CAD build for the part. Positions are in the model's coordinates, mm. A direction names the side the tool comes from. Round coordinates to 2 decimals unless told otherwise and drop trailing zeros. Order: outer loops, then holes, each group sorted by start corner. A loop starts at its lowest first (then second) coordinate and runs counter-clockwise, first axis right, second up. Notation, with made-up numbers: (-32, 73.25) -> (0, 73.25) arc R20 cw to (0, 88.25) -> close; hole circle Ø7 at (12.5, -24.5). An arc over 180 degrees is marked (long way). Answer as CSV lines item,"result". Start each with the question number.
from build123d import *

# Parameters (mm, degrees)
BOSS_EXTRUDE1_DEPTH     = 20
BOSS_EXTRUDE2_DEPTH     = 20
FILLET1_R               = 3
CHAMFER1_SIZE           = 3
FILLET2_R               = 1
CUT_EXTRUDE1_DEPTH      = 71.578127074
CUT_EXTRUDE2_DEPTH      = 2
CUT_EXTRUDE2_DEPTH_BACK = 2
CUT_EXTRUDE2_START      = -10
CHAMFER2_START          = 44.201779004
CHAMFER2_OUTLINE_W      = 6
CHAMFER2_OUTLINE_H      = 20
CHAMFER2_DEPTH          = 1.294789205


with BuildPart() as part:
    # Sketch1 → Boss-Extrude1 (new body)
    with BuildSketch(Plane.XY):
        with BuildLine():
            Line((18, 45.5), (18, 41.407980081))
            Line((18, 41.407980081), (22, 41.407980081))
            Line((22, 41.407980081), (22, 50.5))
            Line((22, 50.5), (-5.5, 50.5))
            Line((-5.5, 50.5), (-5.5, 28.873187411))
            Line((-5.5, 28.873187411), (-5.5, 16.423287813))
            Line((-5.5, 16.423287813), (-0.5, 16.423287813))
            Line((-0.5, 16.423287813), (-0.5, 19))
            Line((-0.5, 19), (5, 19))
            Line((5, 19), (5, 27))
            Line((5, 27), (-0.5, 27))
            Line((-0.5, 27), (-0.5, 44))
            ThreePointArc((-0.5, 44), (-1.560660172, 46.560660172), (1, 45.5))
            Line((1, 45.5), (18, 45.5))
        make_face()
        with BuildLine():
            Line((-5.5, 16.423287813), (-5.5, 28.873187411))
            ThreePointArc((-5.5, 28.873187411), (-9.307611845, 19.680799255), (-18.5, 15.873187411))
            Line((-18.5, 15.873187411), (-21.5, 15.873187411))
            ThreePointArc((-21.5, 15.873187411), (-29.723519433, 18.660367749), (-34.557759664, 25.873187411))
            Line((-34.557759664, 25.873187411), (-39.557759664, 25.873187411))
            ThreePointArc((-39.557759664, 25.873187411), (-33.539294452, 14.749097831), (-21.5, 10.873187411))
            Line((-21.5, 10.873187411), (-18.5, 10.873187411))
            ThreePointArc((-18.5, 10.873187411), (-11.432404679, 12.31875911), (-5.5, 16.423287813))
        make_face()
    extrude(amount=-BOSS_EXTRUDE1_DEPTH)

    # Sketch4 → Boss-Extrude2 (add)
    with BuildSketch(Plane.XY):
        with BuildLine():
            Line((-5.5, 49.330303976), (-5.5, 36.880404378))
            ThreePointArc((-5.5, 36.880404378), (-9.307611845, 46.072792533), (-18.5, 49.880404378))
            Line((-18.5, 49.880404378), (-21.5, 49.880404378))
            ThreePointArc((-21.5, 49.880404378), (-29.723519433, 47.09322404), (-34.557759664, 39.880404378))
            Line((-34.557759664, 39.880404378), (-39.557759664, 39.880404378))
            ThreePointArc((-39.557759664, 39.880404378), (-33.539294452, 51.004493958), (-21.5, 54.880404378))
            Line((-21.5, 54.880404378), (-18.5, 54.880404378))
            ThreePointArc((-18.5, 54.880404378), (-11.432404679, 53.434832679), (-5.5, 49.330303976))
        make_face()
    extrude(amount=-BOSS_EXTRUDE2_DEPTH)

    # Fillet1
    # the kernel refuses this fillet: 3 mm, written as the material it takes off along each edge
    with BuildSketch(Plane(origin=(22, 41.407980081, 7.5), x_dir=(-1, 0, 0), z_dir=(0, 0, -1)), Plane(origin=(22, 50.5, 7.5), x_dir=(0, -1, 0), z_dir=(0, 0, -1))) as fillet1_piece_1:
        with BuildLine():
            CenterArc((FILLET1_R, FILLET1_R), FILLET1_R, 180, 90)
            Line((0, FILLET1_R), (-FILLET1_R * 0.02, FILLET1_R))
            Line((-FILLET1_R * 0.02, FILLET1_R), (-FILLET1_R * 0.02, -FILLET1_R * 0.02))
            Line((-FILLET1_R * 0.02, -FILLET1_R * 0.02), (FILLET1_R, -FILLET1_R * 0.02))
            Line((FILLET1_R, -FILLET1_R * 0.02), (FILLET1_R, 0))
        make_face()
    extrude(amount=35, mode=Mode.SUBTRACT)
    with BuildSketch(Plane(origin=(-5.5, 50.5, 5.942425513), x_dir=(1, 0, 0), z_dir=(0, 0, -1))) as fillet1_piece_2_section:
        with BuildLine():
            CenterArc((2.376970205, 3), FILLET1_R, 217.596829801, 52.403170199)
            Line((0, 1.169696024), (-0.047539404, 1.133089945))
            ThreePointArc((-0.047539404, 1.133089945), (-0.06, 0.584848012), (-0.06, 0))
            Line((-0.06, 0), (0, -0.06))
            Line((0, -0.06), (2.376970205, -0.06))
            Line((2.376970205, -0.06), (2.376970205, 0))
        make_face()
    fillet1_piece_2 = extrude(amount=31.884851026, mode=Mode.PRIVATE)
    fillet1_piece_2 = fillet1_piece_2 - Plane(origin=(-18.5, 36.880404378, 5.942425513), x_dir=(0, 1, 0), z_dir=(0, 0, 1)) * Cylinder(18, 74, mode=Mode.PRIVATE)
    add(fillet1_piece_2, mode=Mode.SUBTRACT)

    # Chamfer1
    chamfer1_edges = [part.edges().sort_by_distance(p)[0] for p in [
        (5, 19, -10),
    ]]
    chamfer(chamfer1_edges, length=CHAMFER1_SIZE)

    # Fillet2
    fillet2_edges = [part.edges().sort_by_distance(p)[0] for p in [
        (-0.5, 16.423287813, -10),
        (1, 45.5, -10),
        (-0.5, 44, -10),
        (-34.557759664, 39.880404378, -10),
        (-39.557759664, 39.880404378, -10),
    ]]
    fillet(fillet2_edges, radius=FILLET2_R)

    # Sketch1<3> → Cut-Extrude1 (cut, through all)
    with BuildSketch(Plane.XY):
        with BuildLine():
            Line((-34.557759664, 25.873187411), (-39.557759664, 25.873187411))
            ThreePointArc((-39.557759664, 25.873187411), (-33.539294452, 14.749097831), (-21.5, 10.873187411))
            Line((-21.5, 10.873187411), (-18.5, 10.873187411))
            ThreePointArc((-18.5, 10.873187411), (-11.432404679, 12.31875911), (-5.5, 16.423287813))
            Line((-5.5, 16.423287813), (-5.5, 28.873187411))
            ThreePointArc((-5.5, 28.873187411), (-9.307611845, 19.680799255), (-18.5, 15.873187411))
            Line((-18.5, 15.873187411), (-21.5, 15.873187411))
            ThreePointArc((-21.5, 15.873187411), (-29.723519433, 18.660367749), (-34.557759664, 25.873187411))
        make_face()
    extrude(amount=-CUT_EXTRUDE1_DEPTH, mode=Mode.SUBTRACT)

    # Sketch3 → Cut-Extrude2 (cut, two sides: drawn at the far end of the back side and taken through both)
    with BuildSketch(Plane.XY.offset(CUT_EXTRUDE2_START - CUT_EXTRUDE2_DEPTH_BACK)):
        with BuildLine():
            ThreePointArc((-10.615862632, 48.696779185), (-12.77767622, 49.881994518), (-15.111856664, 50.675578184))
            Line((-15.111856664, 50.675578184), (-14.837502866, 49.3538207))
            ThreePointArc((-14.837502866, 49.3538207), (-12.420426421, 48.371217451), (-10.248251304, 46.925733813))
            Line((-10.248251304, 46.925733813), (-10.615862632, 48.696779185))
        make_face()
        with BuildLine():
            ThreePointArc((-4.45647435, 39.017159612), (-5.14675526, 41.725731045), (-6.354052632, 44.246699113))
            Line((-6.354052632, 44.246699113), (-6.995300859, 42.933659509))
            ThreePointArc((-6.995300859, 42.933659509), (-5.87936038, 39.99800852), (-5.5, 36.880404378))
            Line((-5.5, 36.880404378), (-4.45647435, 39.017159612))
        make_face()
        with BuildLine():
            ThreePointArc((-21.5, 53.034307539), (-31.973681851, 49.335761876), (-37.80235804, 39.880404378))
            Line((-37.80235804, 39.880404378), (-35.80235804, 39.880404378))
            ThreePointArc((-35.80235804, 39.880404378), (-30.584504262, 47.950694244), (-21.5, 51.085556106))
            Line((-21.5, 51.085556106), (-18.5, 51.085556106))
            ThreePointArc((-18.5, 51.085556106), (-16.793571188, 50.982689168), (-15.111856664, 50.675578184))
            ThreePointArc((-15.111856664, 50.675578184), (-12.77767622, 49.881994518), (-10.615862632, 48.696779185))
            ThreePointArc((-10.615862632, 48.696779185), (-8.240766267, 46.705599481), (-6.354052632, 44.246699113))
            ThreePointArc((-6.354052632, 44.246699113), (-5.14675526, 41.725731045), (-4.45647435, 39.017159612))
            ThreePointArc((-4.45647435, 39.017159612), (-4.418325892, 35.011503653), (-5.5, 31.15446903))
            Line((-5.5, 31.15446903), (-5.5, 28.873187411))
            Line((-5.5, 28.873187411), (-5.5, 27.291421776))
            ThreePointArc((-5.5, 27.291421776), (-4.080428513, 44.162199863), (-18.5, 53.034307539))
            Line((-18.5, 53.034307539), (-21.5, 53.034307539))
        make_face()
    extrude(amount=CUT_EXTRUDE2_DEPTH + CUT_EXTRUDE2_DEPTH_BACK, mode=Mode.SUBTRACT)

    # Chamfer2: read off the stored shape, not the designer's step
    # Chamfer2 outline → Chamfer2 (cut)
    with BuildSketch(Plane(origin=(0, 0, 0), x_dir=(0.8164965809277286, -0.5773502691896223, 0), z_dir=(0.5773502691896223, 0.8164965809277285, 0)).offset(CHAMFER2_START)):
        with Locations((-9, 10)):
            Rectangle(CHAMFER2_OUTLINE_W, CHAMFER2_OUTLINE_H)
    extrude(amount=CHAMFER2_DEPTH, mode=Mode.SUBTRACT)


solid = part.part
Item 1: Tool access for faces 4 (the flat face through (-10.43, 47.8, -10.03)), 5 (the flat face through (-14, 50, -12)), 6 (the cylindrical face through (-9.207, 45.971, -9.86)): list every direction of +Z, -Z, +X, -X, +Y, -Y with a clear straight run to the whole face (end or side of a thin tool).
Item 2: Band-saw the part on B-B, the plane y = 34.5. Give the cut face in (x, z).
Item 3: Band-saw the part on C-C, the plane x = -29. Give the cut face in (y, z).
Item 4: Mould opens along Y. For faces 1 (the flat face through (-38, 39.88, -10)), 2 (the flat face through (5, 24, -10)), 3 (the flat face through (-5, 37.9, -10)) say: released by +Y, released by -Y, zero draft, split by the parting line, or undercut.
Item 5: Probe line 1 (Z direction, x = -21, y = 52); line 2 (X direction, y = 42, z = -18.75); line 3 (Y direction, x = 16, z = -18). List the from-to ranges inside material, lowest first.
Item 6: Pin check, flat tips, straight feed: pin 1 (1.6 mm diameter, centred on x = 3.5, z = -8, fed in from +Y); pin 2 (1 mm diameter, centred on y = 48.5, z = -5, fed in from -X); pin 3 (1.5 mm diameter, centred on x = -20, z = -10, fed in from -Y). Stop position of each tip, or through.
Item 7: Band-saw the part on D-D, the plane z = -10.5. Count the separate pieces of the cut face and the enclosed holes in it, and give its area (3 significant figures).
Values:
1,face 4,"-Y"
1,face 5,"none"
1,face 6,"+Z, -Z, -Y"
2,outline,"(-5.5, -20) -> (-0.5, -20) -> (-0.5, 0) -> (-5.5, 0) -> close; hole (-4.5, -12) -> (-2.52, -12) -> (-2.52, -8) -> (-4.5, -8) -> close"
3,outline,"(47.61, -20) -> (53.71, -20) -> (53.71, 0) -> (47.61, 0) -> close; hole (49.03, -12) -> (51.25, -12) -> (51.25, -8) -> (49.03, -8) -> close"
4,face 1,"released by -Y"
4,face 2,"zero draft"
4,face 3,"undercut"
5,line 1,"-20 to -12, -8 to 0"
5,line 2,"-39.18 to -33.79, -6.55 to -0.5, 19.41 to 20.79"
5,line 3,"45.5 to 50.5"
6,pin 1,"y = 50.5"
6,pin 2,"x = -36.37"
6,pin 3,"y = 49.88"
7,separate pieces,"4"
7,enclosed holes,"0"
7,area,"412 mm²"
